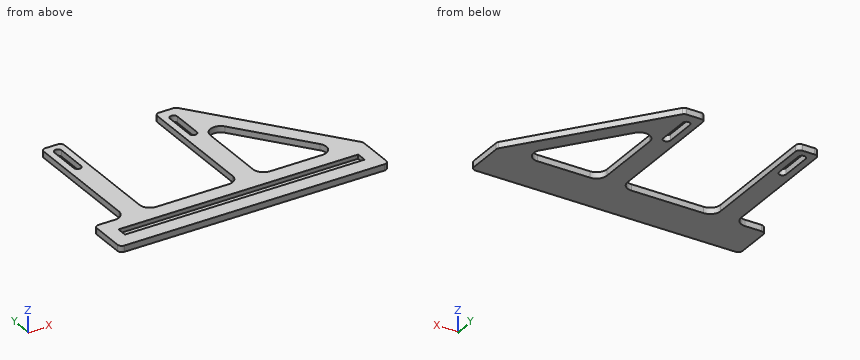
from build123d import *

# Parameters (mm, degrees)
CROQUIS1_W              = 116
CROQUIS1_H              = 5
SALIENTE_EXTRUIR1_DEPTH = 3
CROQUIS1_3_W            = 116
CROQUIS1_3_H            = 5
SALIENTE_EXTRUIR2_DEPTH = 1
REDONDEO1_R             = 5
REDONDEO2_R             = 2


with BuildPart() as part:
    # Croquis1 → Saliente-Extruir1 (new body)
    with BuildSketch(Plane.XY):
        Polygon((-40, 10), (-40, -10), (40, -10), (90, -10), (90, 10), (40, 75), (30, 75), (30, 10), (-15, 10), (-15, 75), (-25, 75), (-25, 10), align=None)
        Polygon((40, 10), (40, 62.6990854), (80.537758, 10), align=None, mode=Mode.SUBTRACT)
        with BuildLine():
            Line((33.25, 68.415525287), (33.25, 53.415525287))
            ThreePointArc((33.25, 53.415525287), (35, 51.665525287), (36.75, 53.415525287))
            Line((36.75, 53.415525287), (36.75, 68.415525287))
            ThreePointArc((36.75, 68.415525287), (35, 70.165525287), (33.25, 68.415525287))
        make_face(mode=Mode.SUBTRACT)
        with Locations((25, 0)):
            Rectangle(CROQUIS1_W, CROQUIS1_H, mode=Mode.SUBTRACT)
        with BuildLine():
            Line((-18.25, 69.952267229), (-18.25, 54.952267229))
            ThreePointArc((-18.25, 54.952267229), (-20, 53.202267229), (-21.75, 54.952267229))
            Line((-21.75, 54.952267229), (-21.75, 69.952267229))
            ThreePointArc((-21.75, 69.952267229), (-20, 71.702267229), (-18.25, 69.952267229))
        make_face(mode=Mode.SUBTRACT)
    extrude(amount=SALIENTE_EXTRUIR1_DEPTH)

    # Croquis1<3> → Saliente-Extruir2 (add)
    with BuildSketch(Plane.XY):
        with Locations((25, 0)):
            Rectangle(CROQUIS1_3_W, CROQUIS1_3_H)
    extrude(amount=SALIENTE_EXTRUIR2_DEPTH)

    # Redondeo1
    redondeo1_edges = [part.edges().sort_by_distance(p)[0] for p in [
        (-25, 10, 1.5),
        (-15, 10, 1.5),
        (30, 10, 1.5),
        (40, 10, 1.5),
        (80.537758, 10, 1.5),
        (40, 62.6990854, 1.5),
    ]]
    fillet(redondeo1_edges, radius=REDONDEO1_R)

    # Redondeo2
    redondeo2_edges = [part.edges().sort_by_distance(p)[0] for p in [
        (-25, 75, 1.5),
        (-15, 75, 1.5),
        (30, 75, 1.5),
        (40, 75, 1.5),
        (90, 10, 1.5),
        (90, -10, 1.5),
        (-40, -10, 1.5),
        (-40, 10, 1.5),
    ]]
    fillet(redondeo2_edges, radius=REDONDEO2_R)


solid = part.part
The listing builds one solid part. Answer for the finished solid, in the listing's coordinates (mm). Round coordinates to 2 decimals unless told otherwise and drop trailing zeros. Loops run counter-clockwise (first coordinate to the right, second up) from the corner with the lowest first, then second, coordinate; pieces in that order, holes last. Notation, with made-up numbers: M -36,71 L -8,71 A24 cw -8,85 Z; hole C 50.25,55.5 d1. An arc over 180 degrees is marked long. Return JSON: item names as keys, results as strings.
Q1. Find section A-A, the plane x = 35. Determine the outline of the cut face in (y, z), plus the area to 4 significant figures.
Results list:
{"outline": "M -10,0 L 51.67,0 L 51.67,3 L 2.5,3 L 2.5,1 L -2.5,1 L -2.5,3 L -10,3 Z; M 70.17,0 L 75,0 L 75,3 L 70.17,3 Z", "area": "189.5 mm2"}
Q2. Find section C-C, the plane x = 20.5. Determine the outline of the cut face in (y, z).
Results list:
{"outline": "M -10,0 L 10,0 L 10,3 L 2.5,3 L 2.5,1 L -2.5,1 L -2.5,3 L -10,3 Z"}
Q3. Each of these flat-tipped pins is pushed along its axis until it touches: pin 1 Ø1.5 at (y, z) = (39, 1) entering from -X; pin 2 Ø1 at (y, z) = (58.5, 0.5) entering from +X; pin 3 Ø1.5 at (y, z) = (29, 0.5) entering from +X; pin 4 Ø8 at (x, y) = (8.5, 15.5) entering from -Z (3 decimals). Where does it stop, or does it pass through?
Results list:
{"pin 1": "stops at x = -25", "pin 2": "stops at x = 53.08", "pin 3": "stops at x = 75.96", "pin 4": "passes through"}
Q4. Find section D-D, the plane y = 56.5. Determine the outline of the cut face in (x, z).
Results list:
{"outline": "M -25,0 L -21.75,0 L -21.75,3 L -25,3 Z; M -18.25,0 L -15,0 L -15,3 L -18.25,3 Z; M 30,0 L 33.25,0 L 33.25,3 L 30,3 Z; M 36.75,0 L 54.23,0 L 54.23,3 L 36.75,3 Z"}
Q5. Find the intervals of material crossed by line 1 along X through (y, z) = (61.5, 1.9); line 2 along Y through (x, z) = (59, 1.7); line 3 along Y through (x, z) = (-20, 1.85), in increasing order. Write a range as from..to.
Results list:
{"line 1": "x = -25..-21.75, -18.25..-15, 30..33.25, 36.75..50.38", "line 2": "y = -10..-2.5, 2.5..10, 38..50.3", "line 3": "y = -10..-2.5, 2.5..53.2, 71.7..75"}
Q6. Find section B-B, the plane y = 12.5. Determine the outline of the cut face in (x, z).
Results list:
{"outline": "M -25.67,0 L -14.33,0 L -14.33,3 L -25.67,3 Z; M 29.33,0 L 40.67,0 L 40.67,3 L 29.33,3 Z; M 74.71,0 L 88.08,0 L 88.08,3 L 74.71,3 Z"}
